Autodesk Inventor part; units mm, degrees
ref_plane "YZ Plane" through (0, 0, 0) normal (1, 0, 0) x (0, 1, 0)
ref_plane "XZ Plane" through (0, 0, 0) normal (0, 1, 0) x (-1, 0, 0)
ref_plane "XY Plane" through (0, 0, 0) normal (0, 0, 1) x (1, 0, 0)
sketch "Sketch1" plane through (0, 0, 0) normal (0, 0, 1) x (1, 0, 0)
  line L0 (0, 0) -> (-156.2246, 0)
  line L1 (-156.2246, 0) -> (-156.2246, -1490)
  line L2 (-156.2246, -1490) -> (0, -1490)
  line L3 (0, -1490) -> (0, 0)
  line L4 (-156.2246, -1390) -> (-66, -1390)
  line L5 (-66, -1390) -> (-66, -1385)
  line L6 (-66, -1385) -> (-156.2246, -1385)
  line L7 (-156.2246, -1385) -> (-156.2246, -1390)
  line L8 (-156.2246, -893.3333) -> (-66, -893.3333)
  line L9 (-66, -893.3333) -> (-66, -888.3333)
  line L10 (-66, -888.3333) -> (-156.2246, -888.3333)
  line L11 (-156.2246, -888.3333) -> (-156.2246, -893.3333)
  line L12 (-156.2246, -396.6667) -> (-66, -396.6667)
  line L13 (-66, -396.6667) -> (-66, -391.6667)
  line L14 (-66, -391.6667) -> (-156.2246, -391.6667)
  line L15 (-156.2246, -391.6667) -> (-156.2246, -396.6667)
  circle A0 centre (-156.2246, -155) radius 30
  point P0 (-156.2246, -391.6667)
  point P1 (-156.2246, -125)
  point P2 (-156.2246, -185)
  dimension "d0" = 1490
  dimension "d1" = 156.2246
  dimension "d2" = 5
  dimension "d4" = 100
  dimension "d7" = 496.6667
  dimension "d23" = 66
  dimension "d28" = 60
  dimension "d29" = 1335
extrude "Plate1" add sketch "Sketch1" along normal blind 4 contours L3 L2 L1 L4 L5 L6 L8 L9 L10 L12 L13 L14 A0 L0
sketch "Sketch2" plane through (4, 0, 0) normal (-1, 0, 0) x (0, -1, 0)
  line L0 (1490, 0) -> (0, 0)
  line L1 (0, 0) -> (0, 60)
  line L2 (0, 60) -> (1490, 60)
  line L3 (1490, 60) -> (1490, 0)
edge flange "Flange1" height 60 angle 90 thickness 4 bend radius 4 thickness toward (-1, 0, 0) relief tear relief width 4 relief depth 2 edges at (0, -745, 4) wall of the first edge with corners at (4, -1490, 0) (4, 0, 0) (4, 0, 60) (4, -1490, 60)
bend "Bend1"
corner "Corner1"
chamfer "Corner Chamfer1" distance 3 angle 45 6 edges at (-156.2246, -1390, 2) (-156.2246, -1385, 2) (-156.2246, -893.3333, 2) (-156.2246, -888.3333, 2) (-156.2246, -391.6667, 2) (-156.2246, -396.6667, 2)
equation "\"d0\" = Стрингер_длина"
equation "\"d1\" = стрингер_глубина_4"
equation "\"d2\" = паз_под_стрингер_толщина"
equation "\"d7\" = Шаг_шпангоутов"
equation "\"d23\" = паз_под_стрингер_глубина - Thickness"
equation "\"d28\" = 2 * радиус_выреза_под_сварку"
equation "\"d12\" = Thickness"
equation "\"d13\" = BendReliefWidth"
equation "\"d14\" = BendReliefDepth"
equation "\"d15\" = MinimumRemnant"
equation "\"d16\" = TransitionRadius"
equation "\"d17\" = ребро_усилителей"
equation "\"d19\" = BendRadius"
equation "\"d20\" = CornerReliefSize"
equation "\"d21\" = GapSize"
equation "\"d22\" = JacobiRadiusSize"
equation "\"BendRadius\" = Thickness"
equation "\"BendReliefWidth\" = Thickness"
equation "\"BendReliefDepth\" = 0.5 * Thickness"
equation "\"CornerReliefSize\" = 4 * Thickness"
equation "\"MinimumRemnant\" = 2 * Thickness"
equation "\"TransitionRadius\" = BendRadius"
equation "\"JacobiRadiusSize\" = BendRadius"
equation "\"GapSize\" = Thickness"
properties part number "GBK 1212 stringer 4" material "Steel"
Can you work these out from the model? Positions are in its coordinate system, mm. A direction names the side the tool comes from. Coordinates: 2 decimals unless noted, no trailing zeros. Order: outer loops, then holes, each group sorted by start corner. A loop starts at its lowest first (then second) coordinate and runs counter-clockwise, first axis right, second up. Notation, with made-up numbers: (46, 88) - (60, 88) arc R18 cw to (60, 110) - close; hole circle Ø3 at (2, 30.5). An arc over 180 degrees is marked (long way). Answer in a Markdown table with one row per item.
1. Suppose I cut it at A-A (x = -87.5). Please give me the cut outline in (y, z).
Reply:
| item | result |
|---|---|
| outline | (-1490, 0) - (-1390, 0) - (-1390, 4) - (-1490, 4) - close; (-1385, 0) - (-893.33, 0) - (-893.33, 4) - (-1385, 4) - close; (-888.33, 0) - (-396.67, 0) - (-396.67, 4) - (-888.33, 4) - close; (-391.67, 0) - (0, 0) - (0, 4) - (-391.67, 4) - close |
2. Suppose I cut it at C-C (x = -140). Please give me the cut outline in (y, z).
Reply:
| item | result |
|---|---|
| outline | (-1490, 0) - (-1390, 0) - (-1390, 4) - (-1490, 4) - close; (-1385, 0) - (-893.33, 0) - (-893.33, 4) - (-1385, 4) - close; (-888.33, 0) - (-396.67, 0) - (-396.67, 4) - (-888.33, 4) - close; (-391.67, 0) - (-180.23, 0) - (-180.23, 4) - (-391.67, 4) - close; (-129.77, 0) - (0, 0) - (0, 4) - (-129.77, 4) - close |
3. For pin 1 (3 mm diameter, centred on x = -130, y = -593, fed in from +Z); pin 2 (1.2 mm diameter, centred on y = -395.5, z = 2.5, fed in from -X), each with a flat end and sliding along its axis, tell me the tip position at first contact or that it passes through.
Reply:
| item | result |
|---|---|
| pin 1 | stops at z = 4 |
| pin 2 | stops at x = -66 |
4. If we mould it in two halves opening along Y, with no side actions, what happens to faces 3 (the cylindrical face through (-126.23, -154.34, 1.97)), 4 (the flat face through (-52, -1490, 3)), 5 (the flat face through (-52, 0, 3)), 6 (the flat face through (4, -735, 34))? For each: pulls with the +Y half, pulls with the -Y half, needs draft (parallel to the pull), parting line crosses it, or undercut.
Reply:
| item | result |
|---|---|
| face 3 | undercut |
| face 4 | pulls with the -Y half |
| face 5 | pulls with the +Y half |
| face 6 | needs draft |
5. Suppose I cut it at B-B (y = -155). Please give me the cut outline in (x, z), and give its area (3 significant figures).
Reply:
| item | result |
|---|---|
| outline | (-126.22, 0) - (-4, 0) arc R8 ccw to (4, 8) - (4, 60) - (0, 60) - (0, 8) arc R4 cw to (-4, 4) - (-126.22, 4) - close |
| area | 735 mm^2 |
6. Suppose I cut it at D-D (z = 19.5). Please give me the cut outline in (x, y).
Reply:
| item | result |
|---|---|
| outline | (0, -1490) - (4, -1490) - (4, 0) - (0, 0) - close |
7. If I drill on line 1 along Z through (x, y) = (-9, -1094.5); line 2 along Z through (x, y) = (-2.5, -861), over which ranges is the centre line in solid material (lowest first)?
Reply:
| item | result |
|---|---|
| line 1 | z = 0 to 4 |
| line 2 | z = 0.14 to 4.29 |
8. For faces 1 (the flat face through (-81, -735, 4)), 2 (the flat face through (-81, -735, 0)), which set-ups out of +Z, -Z, +X, -X, +Y, -Y let a thin tool reach every point of the face, with its end or its side?
Reply:
| item | result |
|---|---|
| face 1 | +Z, -X, +Y, -Y |
| face 2 | -Z, +X, -X, +Y, -Y |
